Design review of the part built by this model. Coordinates are the model's own, in mm. Coordinates: 2 decimals unless noted, no trailing zeros. Loops run counter-clockwise (first coordinate to the right, second up) from the corner with the lowest first, then second, coordinate; pieces in that order, holes last. Notation, with made-up numbers: M 19,48 L 24,48 A14 cw 24,55 Z; hole C 58.25,19.25 d4. An arc over 180 degrees is marked long. One line per item, written item: value.
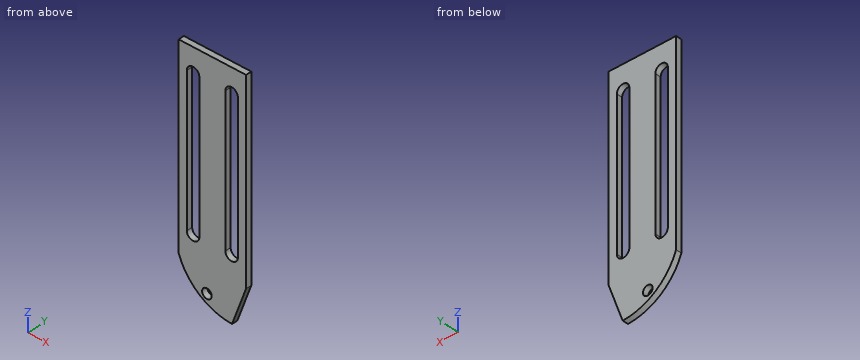
```python
from build123d import *

# Parameters (mm, degrees)
SKETCH1_W           = 35
SKETCH1_H           = 100
SKETCH1_R           = 2.5
BOSS_EXTRUDE1_DEPTH = 3
CUT_EXTRUDE2_DEPTH  = 75.317016198
FILLET1_R           = 30


with BuildPart() as part:
    # Sketch1 → Boss-Extrude1 (new body)
    # profile 1 of 2: a face of its own
    with BuildSketch(Plane(origin=(0, 0, 0), x_dir=(1, 0, 0), z_dir=(0, 1, 0))):
        Rectangle(SKETCH1_W, SKETCH1_H)
    # profile 2 of 2: a face of its own
    with BuildSketch(Plane(origin=(0, 0, 0), x_dir=(1, 0, 0), z_dir=(0, 1, 0))):
        Polygon((17.5, 50), (10.220595315, 70), (-24.779404685, 70), (-17.5, 50), align=None)
        with Locations(Location((-2.830309398, 62, 0), (0, 0, 270))):
            Circle(SKETCH1_R, mode=Mode.SUBTRACT)
    extrude(amount=BOSS_EXTRUDE1_DEPTH)

    # Sketch3 → Cut-Extrude2 (cut, through all)
    with BuildSketch(Plane(origin=(0, 3, 0), x_dir=(1, 0, 0), z_dir=(0, 1, 0))):
        with BuildLine():
            Line((-13.25, -37.5), (-13.25, 37.5))
            ThreePointArc((-13.25, 37.5), (-10, 40.75), (-6.75, 37.5))
            Line((-6.75, 37.5), (-6.75, -37.5))
            ThreePointArc((-6.75, -37.5), (-10, -40.75), (-13.25, -37.5))
        make_face()
        with BuildLine():
            Line((6.75, -37.5), (6.75, 37.5))
            ThreePointArc((6.75, 37.5), (10, 40.75), (13.25, 37.5))
            Line((13.25, 37.5), (13.25, -37.5))
            ThreePointArc((13.25, -37.5), (10, -40.75), (6.75, -37.5))
        make_face()
    extrude(amount=-CUT_EXTRUDE2_DEPTH, mode=Mode.SUBTRACT)

    # Fillet1
    # the kernel refuses this fillet: 30 mm, written as the material it takes off along each edge
    with BuildSketch(Plane(origin=(-24.779404685, -88.909189832, -70), x_dir=(1, 0, 0), z_dir=(0, 1, 0))) as fillet1_piece_1:
        with BuildLine():
            CenterArc((35.563675933, -30), FILLET1_R, 90, 70.528779366)
            Line((7.279404685, -20), (0, 0))
            Line((0, 0), (35.563675933, 0))
        make_face()
    extrude(amount=180.818379664, mode=Mode.SUBTRACT)


solid = part.part
```
(1) To check wall thickness, follow line 1 along X through (y, z) = (2.5, 19.5); line 2 along Z through (x, y) = (9, 1.75); line 3 along Z through (x, y) = (-1.5, 2.3). State the ranges of each line that lie inside material, in increasing order. Write a range as [from, to].
Reply:
line 1: x = [-17.5, -13.25], [-6.75, 6.75], [13.25, 17.5]
line 2: z = [-69.95, -40.59], [40.59, 50]
line 3: z = [-67.37, -64.12], [-59.88, 50]
(2) We need section D-D on z = -62. State the section outline as (x, y) points, then the cut area to 3 significant figures.
Reply:
outline: M -9.61,0 L -5.33,0 L -5.33,3 L -9.61,3 Z; M -0.33,0 L 13.13,0 L 13.13,3 L -0.33,3 Z
area: 53.2 mm2
(3) We need section A-A on z = -36. State the section outline as (x, y) points.
Reply:
outline: M -17.5,0 L -13.25,0 L -13.25,3 L -17.5,3 Z; M -6.75,0 L 6.75,0 L 6.75,3 L -6.75,3 Z; M 13.25,0 L 17.5,0 L 17.5,3 L 13.25,3 Z
(4) We need section B-B on x = -10. State the section outline as (y, z) points, then the cut area to 3 significant figures.
Reply:
outline: M 0,-61.63 L 3,-61.63 L 3,-40.75 L 0,-40.75 Z; M 0,40.75 L 3,40.75 L 3,50 L 0,50 Z
area: 90.4 mm2
(5) We need section C-C on y = 1.7. State the section outline as (x, z) points.
Reply:
outline: M -17.5,-50 A30 ccw 10.22,-69.99 L 17.5,-50 L 17.5,50 L -17.5,50 Z; hole M -13.25,-37.5 A3.25 ccw -6.75,-37.5 L -6.75,37.5 A3.25 ccw -13.25,37.5 Z; hole C -2.83,-62 d5; hole M 6.75,-37.5 A3.25 ccw 13.25,-37.5 L 13.25,37.5 A3.25 ccw 6.75,37.5 Z
